```python
from build123d import *

# Parameters (mm, degrees)
BOSS_EXTRUDE1_DEPTH = 10
CIRPATTERN1_COUNT   = 2
CIRPATTERN1_ANGLE   = 90
SKETCH4_R           = 2
SKETCH4_R_2         = 11
BOSS_EXTRUDE2_DEPTH = 3


with BuildPart() as part:
    # Sketch1 → Boss-Extrude1 (new body)
    with BuildSketch(Plane(origin=(0, 0, 0), x_dir=(1, 0, 0), z_dir=(0, 1, 0))):
        with BuildLine():
            Line((0, 15), (-26.900155428, 6.278700475))
            Line((-26.900155428, 6.278700475), (-37.47437809, 2.750369919))
            Line((-37.47437809, 2.750369919), (-36.958650594, -0.903972442))
            Line((-36.958650594, -0.903972442), (-26.900155428, 3.317423045))
            Line((-26.900155428, 3.317423045), (-2.821131559, 11.193160892))
            ThreePointArc((-2.821131559, 11.193160892), (11.303828334, 2.338610491), (1.8517881, -11.393705054))
            Line((1.8517881, -11.393705054), (-25.145499842, -12.903972442))
            Line((-25.145499842, -12.903972442), (-32.586903668, -12.903972442))
            Line((-32.586903668, -12.903972442), (-36.958650594, -12.903972442))
            Line((-36.958650594, -12.903972442), (-36.958650594, -15.903972442))
            Line((-36.958650594, -15.903972442), (-0.325723138, -14.996463064))
            ThreePointArc((-0.325723138, -14.996463064), (14.99911574, -0.16287117), (0, 15))
        make_face()
    boss_extrude1 = extrude(amount=BOSS_EXTRUDE1_DEPTH)

    # CirPattern1: Boss-Extrude1 ×2 about axis
    cirpattern1_axis = Axis((-31.052075218, 5, 0), (0, 0, -1))
    for i in range(1, CIRPATTERN1_COUNT):
        add(boss_extrude1.rotate(cirpattern1_axis, i * CIRPATTERN1_ANGLE / (CIRPATTERN1_COUNT - 1)))

    # Sketch4 → Boss-Extrude2 (add)
    with BuildSketch(Plane(origin=(0, 0, 12.903972442), x_dir=(-1, 0, 0), z_dir=(0, 0, -1))):
        Polygon((25.145499842, 5), (29.375972464, -0.906575376), (6.490188193, -17.298084434), (19.427171172, -35.360667965), (-10.945093119, -57.114226389), (-34.236490518, -24.59483514), (-3.864226227, -2.841276715), (2.259715572, -11.391509058), align=None)
        with Locations((-4.040125025, -10.790378208)):
            Circle(SKETCH4_R, mode=Mode.SUBTRACT)
        with Locations((11.099283284, -31.92798252)):
            Circle(SKETCH4_R, mode=Mode.SUBTRACT)
        with Locations((-25.189607513, -27.394689404)):
            Circle(SKETCH4_R, mode=Mode.SUBTRACT)
        with Locations((-9.336361168, -48.002323435)):
            Circle(SKETCH4_R, mode=Mode.SUBTRACT)
        with Locations((-7.525518654, -29.277184542)):
            Circle(SKETCH4_R_2, mode=Mode.SUBTRACT)
    extrude(amount=-BOSS_EXTRUDE2_DEPTH)


solid = part.part
```
Verification items for the finished model (mm, model axes). A direction names the side the tool comes from. Round coordinates to 2 decimals unless told otherwise and drop trailing zeros. Order: outer loops, then holes, each group sorted by start corner. A loop starts at its lowest first (then second) coordinate and runs counter-clockwise, first axis right, second up. Notation, with made-up numbers: (-21.75, -34.75) - (-0.75, -34.75) arc R15 ccw to (-0.75, -18.75) - close; hole circle Ø3 at (19, 65.5). An arc over 180 degrees is marked (long way). Use CSV: the item, a comma, the result in double quotes.
(1) Section check D-D on z = 10.5. Record the boundary of the cut face in (x, y).
Entries:
outline,"(-36.05, -36.76) - (-26.05, -36.76) - (-26.05, -30.85) - (-36.05, -30.85) - close; (4.8, 0) - (10.71, 0) - (10.71, 10) - (4.8, 10) - close"
(2) Thickness scan on probe 1 along Y at (x, z) = (-13, -8); probe 2 along Y at (x, z) = (11, 13.5); probe 3 along Z at (x, y) = (-8, -31). Record the ranges inside material, lowest first. Write a range as from..to.
Entries:
probe 1,"0..10"
probe 2,"-57.04..-49.11, -46.89..-39.71, -18.84..-7.95"
probe 3,"12.9..15.9"
(3) Mould release check, pull along Y, two halves, no side actions. Record for faces 1 (the face through (4.474, -12.743, 14.383)), 2 (the face through (-37.22, 4.93, -0.95)), 3 (the face through (-32.557, 4.343, -5.113)): released by +Y, released by -Y, zero draft, split by the parting line, or undercut.
Entries:
face 1,"undercut"
face 2,"zero draft"
face 3,"released by +Y"
(4) Section check A-A on z = 6.5. Record the boundary of the cut face in (x, y), and give its area (3 significant figures).
Entries:
outline,"(-36.05, -39.57) - (-26.05, -39.57) - (-26.05, -35.59) - (-36.05, -35.59) - close; (9.54, 0) - (13.52, 0) - (13.52, 10) - (9.54, 10) - close"
area,"79.6 mm^2"
(5) Access from +Z, -Z, +X, -X, +Y, -Y to the whole of each face (thin tool, end or side, straight path). Record for faces 4 (the face through (-31.12, -14.59, 12.14)), 5 (the face through (-33, 0, -2)), 6 (the face through (-26.052, 7, -2)), 7 (the face through (-31, 10.907, 14)).
Entries:
face 4,"+X, -X, +Y"
face 5,"+X, -X"
face 6,"+Y, -Y"
face 7,"+Z, +X, -X, +Y"
(6) Section check B-B on y = -14.5. Record the boundary of the cut face in (x, z), and give its area (3 significant figures).
Entries:
outline,"(-36.05, -11.25) - (-26.05, -11.25) - (-26.05, -8.34) - (-36.05, -8.34) - close; (-36.05, 12.14) - (-26.05, 12.14) - (-26.05, 15.27) - (-36.05, 15.27) - close; (-10.4, 12.9) - (20.14, 12.9) - (20.14, 15.9) - (-10.4, 15.9) - close"
area,"152 mm^2"
(7) Gauge pin test, flat ends, axial feed: pin 1 Ø20.5 at (x, y) = (1.5, -26) entering from -Z; pin 2 Ø10 at (x, z) = (-9.5, 0) entering from -Y; pin 3 Ø1.3 at (x, z) = (-34, -1) entering from -Y; pin 4 Ø10 at (x, z) = (3, 6) entering from -Y. Record the tip position at first contact, or that the pin passes through.
Entries:
pin 1,"z = 12.9"
pin 2,"through"
pin 3,"y = -41.05"
pin 4,"y = 0"
